Design review of the part built by this model. Coordinates are the model's own, in mm. Round coordinates to 2 decimals unless told otherwise and drop trailing zeros. Write each loop counter-clockwise with the first axis right and the second up, starting at its lowest first coordinate (ties: lowest second). Pieces come first, ordered by that corner, then holes. Notation, with made-up numbers: (9, -29.75) -> (35, -29.75) arc R20 cw to (35, 6.25) -> close; hole circle Ø5 at (7.5, -6). An arc over 180 degrees is marked (long way). Write item = value, one per line. Start each with the question number.
Item 1: Add section A-A, the plane x = -205.5. State the section outline as (y, z) points.
Item 2: For pin 1 Ø4 at (x, y) = (-221, -12) entering from +Z; pin 2 Ø12 at (x, y) = (-170, -3.5) entering from -Z; pin 3 Ø3 at (y, z) = (8.5, 297.5) entering from +X, all flat-tipped, find the tip position at first contact; note any pin that passes through.
Item 3: Add section B-B, the plane z = 1032. State the section outline as (x, y) points, then the cut area to 3 significant figures.
Item 4: Add section C-C, the plane x = -340.5. State the section outline as (y, z) points, then the cut area to 3 significant figures.
Item 5: To check wall thickness, follow L1, parallel to Y at x = 0, z = 1134; L2, parallel to X at y = 0, z = 823. State the ranges of each line that lie inside material, in increasing order.
Autodesk Inventor part; units mm, degrees
ref_plane "Work Plane4" through (0, 0, 249) normal (0, 0, 1) x (1, 0, 0)
ref_plane "Work Plane5" through (0, 0, 249) normal (0, 0, 1) x (1, 0, 0)
ref_plane "YZ Plane" through (0, 0, 0) normal (1, 0, 0) x (0, 1, 0)
sketch "Sketch1" plane through (0, 0, 0) normal (0, 0, 1) x (1, 0, 0)
  circle A0 centre (0, 0) radius 11
  circle A1 centre (0, 0) radius 9
  dimension "d9" = 22
  dimension "d40" = 18
extrude "mast" add sketch "Sketch1" along normal blind 1310 and the other way blind 275
sketch "Sketch4" plane through (0, 0, 0) normal (1, 0, 0) x (0, 1, 0)
  circle A0 centre (0, 818) radius 11
  circle A1 centre (0, 260) radius 11
  line L0 (-20.25, 247.25) -> (20.25, 247.25)
  line L1 (20.25, 247.25) -> (20.25, 272.75)
  line L2 (20.25, 272.75) -> (-20.25, 272.75)
  line L3 (-20.25, 272.75) -> (-20.25, 247.25)
  line L4 (-20.25, 247.25) -> (20.25, 272.75) construction
  line L5 (20.25, 247.25) -> (-20.25, 272.75) construction
  line L6 (-20.25, 805.25) -> (20.25, 805.25)
  line L7 (20.25, 805.25) -> (20.25, 830.75)
  line L8 (20.25, 830.75) -> (-20.25, 830.75)
  line L9 (-20.25, 830.75) -> (-20.25, 805.25)
  line L10 (-20.25, 805.25) -> (20.25, 830.75) construction
  line L11 (20.25, 805.25) -> (-20.25, 830.75) construction
  point P0 (0, 0)
  dimension "d19" = 22
  dimension "d20" = 818
  dimension "d21" = 22
  dimension "d22" = 260
  dimension "d97" = 40.5
  dimension "d98" = 25.5
  dimension "d99" = 40.5
  dimension "d100" = 25.5
extrude "tail" add sketch "Sketch4" against normal blind 240 contours A0 | A1
sketch "Sketch8" plane through (-240, 0, 260) normal (-1, 0, 0) x (0, 0, 1)
  circle A0 centre (0, 0) radius 11
  circle A1 centre (0, 0) radius 11
  circle A2 centre (0, 0) radius 9
  circle A3 centre (558, 0) radius 11
  circle A4 centre (558, 0) radius 9
  dimension "d42" = 18
  dimension "d52" = 18
extrude "tail2" add sketch "Sketch8" along normal blind 180 contours A2 | A4
ref_plane "Work Plane4" through (0, 0, 249) normal (0, 0, 1) x (1, 0, 0)
sketch "Sketch11" plane through (-420, 0, 818) normal (-1, 0, 0) x (0, 0, 1)
  circle A0 centre (0, 0) radius 9
  circle A1 centre (-558, 0) radius 11
  circle A2 centre (0, 0) radius 11
  circle A3 centre (0, 0) radius 7
  circle A4 centre (-558, 0) radius 9
  point P0 (-818, 0)
  dimension "d53" = 22
  dimension "d54" = 22
  dimension "d58" = 14
extrude "tail3" add sketch "Sketch11" along normal blind 30 contours A0 | A1 | A2 | A3 | A4
ref_plane "Work Plane5" through (0, 0, 249) normal (0, 0, 1) x (1, 0, 0)
sketch "Sketch20" plane through (0, 0, 249) normal (0, 0, 1) x (1, 0, 0)
  circle A0 centre (-435, 0) radius 4
  line L0 (-450, 11) -> (-450, -11)
  line L1 (-450, 0) -> (-430, 0) construction
  point P0 (0, 0)
  dimension "d82" = 8
  dimension "d83" = 15
extrude "tail holes" cut sketch "Sketch20" along normal through all
sketch "Sketch14" plane through (0, 0, 260) normal (1, 0, 0) x (0, 1, 0)
  circle A0 centre (0, 558) radius 11
  circle A1 centre (0, 0) radius 11
  point P0 (0, -260)
extrude "weight" add sketch "Sketch14" along normal blind 120
sketch "Sketch21" plane through (120, 0, 260) normal (1, 0, 0) x (0, 0, -1)
  circle A0 centre (0, 0) radius 11
  circle A1 centre (0, 0) radius 9
  circle A2 centre (-558, 0) radius 11
  circle A3 centre (-558, 0) radius 9
  point P0 (260, 0)
  dimension "d88" = 18
  dimension "d89" = 18
extrude "weight2" add sketch "Sketch21" along normal blind 250 contours A1 | A3
extrude "reinforcement tube" add sketch "Sketch4" along normal mid plane 140
equation "\"tail_height\" = 530"
properties part number "sail_skeleton2"
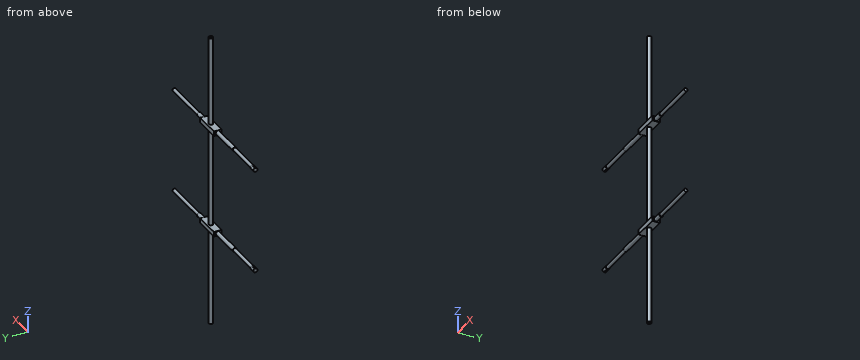
Result set:
q1.outline = circle Ø22 at (0, 260); circle Ø22 at (0, 818)
q2.pin_1 = 822.58
q2.pin_2 = 249
q2.pin_3 = 8.49
q3.outline = circle Ø22 at (0, 0); hole circle Ø18 at (0, 0)
q3.area = 126 mm²
q4.outline = circle Ø18 at (0, 260); circle Ø18 at (0, 818)
q4.area = 509 mm²
q5.L1 = -11 to -9, 9 to 11
q5.L2 = -450 to -439, -431 to 370
